Model file for the job. Use its own axes, mm. A direction names the side the tool comes from. Coordinates: 2 decimals unless noted, no trailing zeros. Write each loop counter-clockwise with the first axis right and the second up, starting at its lowest first coordinate (ties: lowest second). Pieces come first, ordered by that corner, then holes.
Q1. Which spindle directions (+Z, -Z, +X, -X, +Y, -Y) get a long thin tool onto all of the face, cutting with end or side? Do faces 1 (the flat face through (-11, 46, -39.688)), 2 (the cylindrical face through (7.03, 68.56, -43.31)). Say none if no direction does.
Q2. Band-saw the part on D-D, the plane x = 0. Write the cut outline in (y, z).
Q3. Pull direction X, two halves, no side cores. Call faces 3 (the flat face through (1.41, 31.12, 43.31)), 4 (the flat face through (-21, 93.662, -21)): released by +X, released by -X, zero draft, split by the parting line, or undercut.
Q4. Band-saw the part on B-B, the plane z = 37.5. Write the cut outline in (x, y).
Q5. Band-saw the part on C-C, the plane z = 0. Write the cut outline in (x, y), plus the area to 3 significant figures.
Q6. Drill centre lines: probe 1 along Y at (x, z) = (-32.5, -4); probe 2 along Z at (x, y) = (-31.5, 66.5); probe 3 along X at (y, z) = (89.5, 0). Where is each one in solid material? Low to high.
Q7. Band-saw the part on A-A, the plane y = 85. Write the cut outline in (x, z), plus the area to 3 significant figures.
from build123d import *

# Parameters (mm, degrees)
SKETCH1_W           = 93.6625
SKETCH1_H           = 93.6625
BOSS_EXTRUDE1_DEPTH = 93.6625
SKETCH3_R           = 26.9875
CUT_EXTRUDE1_DEPTH  = 115.712666517
SKETCH4_W           = 79.375
SKETCH4_H           = 79.375
CUT_EXTRUDE2_DEPTH  = 141.49375
CUT_EXTRUDE3_DEPTH  = 141.49375
FILLET1_R           = 1.5
FILLET2_R           = 1.5


with BuildPart() as part:
    # Sketch1 → Boss-Extrude1 (new body)
    with BuildSketch(Plane(origin=(0, 0, 0), x_dir=(1, 0, 0), z_dir=(0, 1, 0))):
        Rectangle(SKETCH1_W, SKETCH1_H)
    extrude(amount=BOSS_EXTRUDE1_DEPTH)

    # Sketch3 → Cut-Extrude1 (cut, through all)
    with BuildSketch(Plane(origin=(0, 93.6625, 0), x_dir=(1, 0, 0), z_dir=(0, 1, 0))):
        with Locations(Location((0, 0, 0), (0, 0, 270))):
            Circle(SKETCH3_R)
    extrude(amount=-CUT_EXTRUDE1_DEPTH, mode=Mode.SUBTRACT)

    # Sketch4 → Cut-Extrude2 (cut, through all)
    with BuildSketch(Plane.ZY.offset(46.83125)):
        with Locations((0, 46.83125)):
            Rectangle(SKETCH4_W, SKETCH4_H)
    extrude(amount=-CUT_EXTRUDE2_DEPTH, mode=Mode.SUBTRACT)

    # Sketch5 → Cut-Extrude3 (cut, through all)
    with BuildSketch(Plane.XY.offset(46.83125)):
        Polygon((26.19375, 46.83125), (8.094313896, 52.712113281), (8.094313896, 71.742986624), (-3.091752793, 56.346686671), (-21.191188896, 62.227549952), (-10.005122207, 46.83125), (-21.191188896, 31.434950048), (-3.091752793, 37.315813329), (8.094313896, 21.919513376), (8.094313896, 40.950386719), align=None)
    extrude(amount=-CUT_EXTRUDE3_DEPTH, mode=Mode.SUBTRACT)

    # Fillet1
    fillet1_edges = [part.edges().sort_by_distance(p)[0] for p in [
        (26.19375, 46.83125, 43.259375),
        (8.094313896, 40.950386719, 43.259375),
        (8.094313896, 21.919513376, 43.259375),
        (-3.091752793, 37.315813329, 43.259375),
        (-21.191188896, 31.434950048, 43.259375),
        (-10.005122207, 46.83125, 43.259375),
        (-21.191188896, 62.227549952, 43.259375),
        (-3.091752793, 56.346686671, 43.259375),
        (8.094313896, 71.742986624, 43.259375),
        (8.094313896, 52.712113281, 43.259375),
    ]]
    fillet(fillet1_edges, radius=FILLET1_R)

    # Fillet2
    fillet2_edges = [part.edges().sort_by_distance(p)[0] for p in [
        (26.19375, 46.83125, -43.259375),
        (8.094313896, 40.950386719, -43.259375),
        (8.094313896, 21.919513376, -43.259375),
        (-3.091752793, 37.315813329, -43.259375),
        (-21.191188896, 31.434950048, -43.259375),
        (-10.005122207, 46.83125, -43.259375),
        (-21.191188896, 62.227549952, -43.259375),
        (-3.091752793, 56.346686671, -43.259375),
        (8.094313896, 71.742986624, -43.259375),
        (8.094313896, 52.712113281, -43.259375),
    ]]
    fillet(fillet2_edges, radius=FILLET2_R)


solid = part.part
Answer sheet:
1. face 1: +X, -X
1. face 2: +Z, -Z
2. outline: (0, -46.83) - (33.06, -46.83) - (33.06, -39.69) - (7.14, -39.69) - (7.14, -26.99) - (0, -26.99) - close; (0, 26.99) - (7.14, 26.99) - (7.14, 39.69) - (33.06, 39.69) - (33.06, 46.83) - (0, 46.83) - close; (60.6, -46.83) - (93.66, -46.83) - (93.66, -26.99) - (86.52, -26.99) - (86.52, -39.69) - (60.6, -39.69) - close; (60.6, 39.69) - (86.52, 39.69) - (86.52, 26.99) - (93.66, 26.99) - (93.66, 46.83) - (60.6, 46.83) - close
3. face 3: undercut
3. face 4: zero draft
4. outline: (-46.83, 0) - (46.83, 0) - (46.83, 7.14) - (-46.83, 7.14) - close; (-46.83, 86.52) - (46.83, 86.52) - (46.83, 93.66) - (-46.83, 93.66) - close
5. outline: (-46.83, 0) - (-26.99, 0) - (-26.99, 7.14) - (-46.83, 7.14) - close; (-46.83, 86.52) - (-26.99, 86.52) - (-26.99, 93.66) - (-46.83, 93.66) - close; (26.99, 0) - (46.83, 0) - (46.83, 7.14) - (26.99, 7.14) - close; (26.99, 86.52) - (46.83, 86.52) - (46.83, 93.66) - (26.99, 93.66) - close
5. area: 567 mm2
6. probe 1: y = 0 to 7.14, 86.52 to 93.66
6. probe 2: z = -46.83 to -39.69, 39.69 to 46.83
6. probe 3: x = -46.83 to -26.99, 26.99 to 46.83
7. outline: (-46.83, -46.83) - (46.83, -46.83) - (46.83, -39.69) - (-46.83, -39.69) - close; (-46.83, 39.69) - (46.83, 39.69) - (46.83, 46.83) - (-46.83, 46.83) - close
7. area: 1,340 mm2
